Build history of the part. All positions in model axes, mm. Face numbers are marked on the shaded views. Give positions to 0.01 mm unless a question says otherwise; leave off trailing zeros. Order: outer loops, then holes, each group sorted by start corner. A loop starts at its lowest first (then second) coordinate and runs counter-clockwise, first axis right, second up. Notation, with made-up numbers: (13, -7.5) -> (57, -7.5) arc R34 ccw to (57, 23.5) -> close; hole circle Ø11 at (38, 1.5). An arc over 180 degrees is marked (long way). One line per item, written item: value. Start each with the question number.
(1) Pin check, flat tips, straight feed: pin 1 (2 mm diameter, centred on x = -12, z = 31, fed in from -Y); pin 2 (2.5 mm diameter, centred on x = 0, y = 0, fed in from -Z) (3 decimals); pin 3 (4 mm diameter, centred on x = -5.5, y = -1, fed in from -Z). Stop position of each tip, or through.
(2) Saw through at A-A on z = 28.5. Give the cut face in (x, y), plus the area to 3 significant figures.
(3) Saw through at B-B on z = 18. Give the cut face in (x, y).
(4) Probe line 1 (Y direction, x = 0, z = 52.25); line 2 (X direction, y = 0, z = 7.5); line 3 (Y direction, x = 0, z = 13.75). List the from-to ranges inside material, lowest first.
(5) Saw through at C-C on z = 35.5. Give the cut face in (x, y), plus the area to 3 significant figures.
(6) Two-plate mould, pull along X, no slides. Class the marked faces 1, 2 and 3: +X half, -X half, draft (parallel to the pull), parting line (faces both ways), or undercut.
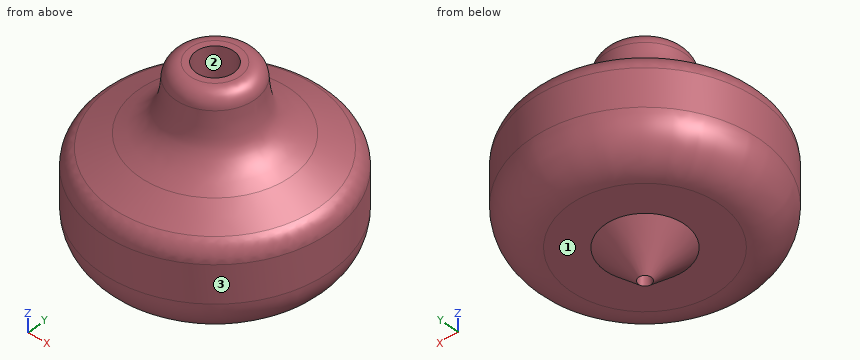
```python
from build123d import *

# Parameters (mm, degrees)
F2_R     = 10.16
F3_R     = 5.08
F4_R     = 4.76885
F5_DEPTH = 11.43
F6_R     = 1.6002
F7_DEPTH = 19.685
F8_R     = 3.81


# Not quite as in the source:
# - a fillet or chamfer that OpenCascade refuses, or shapes differently, is made with other operations: its cross-section is extruded or revolved along the edge and cut away or added


with BuildPart() as f1:
    # F0 (on Front) → F1 (revolve)
    with BuildSketch(Plane.XZ):
        Polygon((0, 54.61), (0, 0), (10.16, 9.5882897328), (29.21, 9.5882897328), (29.21, 32.4482897328), (10.16, 41.9100038707), (10.16, 54.61), align=None)
    revolve(axis=Axis((0, 0, 27.305), (0, 0, 1)))

    # F2
    f2_edges = [f1.edges().sort_by_distance(p)[0] for p in [
        (-29.21, 0, 9.58829),
    ]]
    fillet(f2_edges, radius=F2_R)

    # F3
    f3_edges = [f1.edges().sort_by_distance(p)[0] for p in [
        (-29.21, 0, 32.44829),
    ]]
    fillet(f3_edges, radius=F3_R)

    # F4 (on face) → F5 (cut)
    with BuildSketch(Plane.XY.offset(54.61)):
        Circle(F4_R)
    extrude(amount=-F5_DEPTH, mode=Mode.SUBTRACT)

    # F6 (on Top) → F7 (cut)
    with BuildSketch(Plane.XY):
        Circle(F6_R)
    extrude(amount=F7_DEPTH, mode=Mode.SUBTRACT)

    # F8
    f8_edges = [f1.edges().sort_by_distance(p)[0] for p in [
        (-10.16, 0, 54.61),
    ]]
    fillet(f8_edges, radius=F8_R)

    # F9: fillet of radius 16.51 on 3 edges, made by hand

    # F9_s1 → F9_t2 (revolve)
    with BuildSketch(Plane.XZ):
        with BuildLine():
            add(Edge.make_bspline(
                [(10.1513687758, 51.056311199), (10.7891371387, 41.5975253532), (19.279794422, 37.3804034604)],
                knots=[0, 0, 0, 1, 1, 1], degree=2, weights=[1, 1.8571428571, 1]))
            Line((19.279794422, 37.3804034604), (18.5453771838, 35.9017445003))
            Line((18.5453771838, 35.9017445003), (9.4255827618, 40.4313449106))
            Line((9.4255827618, 40.4313449106), (8.509, 41.9100038707))
            ThreePointArc((8.509, 41.9100038707), (8.509, 50.8), (8.5041089729, 50.9452430127))
            Line((8.5041089729, 50.9452430127), (10.1513687758, 51.056311199))
        make_face()
    revolve(axis=Axis((0, 0, 41.9100038707), (0, 0, 1)))


solid = f1.part
```
Results below:
1. pin 1: stops at y = -26.85
1. pin 2: stops at z = 19.685
1. pin 3: stops at z = 3.39
2. outline: circle Ø58.42 at (0, 0)
2. area: 2,680 mm²
3. outline: circle Ø58.12 at (0, 0); hole circle Ø3.2 at (0, 0)
4. line 1: y = -9.87 to -4.77, 4.77 to 9.87
4. line 2: x = -7.95 to -1.6, 1.6 to 7.95
4. line 3: y = -27.25 to -1.6, 1.6 to 27.25
5. outline: circle Ø46.13 at (0, 0)
5. area: 1,670 mm²
6. face 1: draft
6. face 2: undercut
6. face 3: parting line
